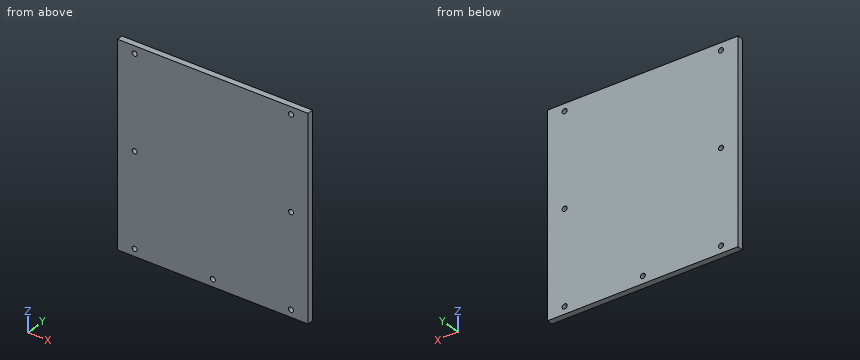
from build123d import *

# Parameters (mm, degrees)
SKETCH2_W           = 190.5
SKETCH2_H           = 203.2
BOSS_EXTRUDE1_DEPTH = 6
SKETCH5_R           = 2.5
CUT_EXTRUDE6_DEPTH  = 7


with BuildPart() as part:
    # Sketch2 → Boss-Extrude1 (new body)
    with BuildSketch(Plane(origin=(0, 0, 0), x_dir=(1, 0, 0), z_dir=(0, 1, 0))):
        Rectangle(SKETCH2_W, SKETCH2_H)
    extrude(amount=BOSS_EXTRUDE1_DEPTH)

    # Sketch5 → Cut-Extrude6 (cut, through all)
    with BuildSketch(Plane(origin=(0, 6, 0), x_dir=(1, 0, 0), z_dir=(0, 1, 0))):
        with Locations((-78.187036158, 94.165073798)):
            Circle(SKETCH5_R)
        with Locations((0, 94.165073798)):
            Circle(SKETCH5_R)
        with Locations((78.187036158, 0)):
            Circle(SKETCH5_R)
        with Locations((-78.187036158, 0)):
            Circle(SKETCH5_R)
        with Locations((78.187036158, 94.165073798)):
            Circle(SKETCH5_R)
        with Locations((-78.187036158, -94.165073798)):
            Circle(SKETCH5_R)
        with Locations((78.187036158, -94.165073798)):
            Circle(SKETCH5_R)
    extrude(amount=-CUT_EXTRUDE6_DEPTH, mode=Mode.SUBTRACT)


solid = part.part
For this review, take the finished solid that the model builds, in its own axes (mm). Give positions to 0.01 mm unless a question says otherwise; leave off trailing zeros. Order: outer loops, then holes, each group sorted by start corner. A loop starts at its lowest first (then second) coordinate and runs counter-clockwise, first axis right, second up. Notation, with made-up numbers: (36.5, 23) -> (80.5, 23) arc R15 cw to (80.5, 28) -> close; hole circle Ø8 at (74, 43). An arc over 180 degrees is marked (long way). Write item = value, one per line.
1) We need section B-B, the plane x = 0. Give the boundary of the cut face in (y, z).
Findings:
outline = (0, -101.6) -> (6, -101.6) -> (6, -96.67) -> (0, -96.67) -> close; (0, -91.67) -> (6, -91.67) -> (6, 101.6) -> (0, 101.6) -> close
2) We need section A-A, the plane z = 0. Give the boundary of the cut face in (x, y).
Findings:
outline = (-95.25, 0) -> (-80.69, 0) -> (-80.69, 6) -> (-95.25, 6) -> close; (-75.69, 0) -> (75.69, 0) -> (75.69, 6) -> (-75.69, 6) -> close; (80.69, 0) -> (95.25, 0) -> (95.25, 6) -> (80.69, 6) -> close
3) Insertion check: pin 1 (4.5 mm diameter, centred on x = 78.19, z = 94.17, fed in from +Y). The pin has a flat end and moves straight along its axis. Give the tip position at first contact, or say it passes through.
Findings:
pin_1 = through
4) To check wall thickness, follow L1, parallel to X at y = 3.85, z = 0; L2, parallel to Z at x = -77.5, y = 4.5; L3, parallel to Z at x = 1, y = 4.05. State the ranges of each line that lie inside material, in increasing order. Write a range as from..to.
Findings:
L1 = -95.25..-80.69, -75.69..75.69, 80.69..95.25
L2 = -101.6..-96.57, -91.76..-2.4, 2.4..91.76, 96.57..101.6
L3 = -101.6..-96.46, -91.87..101.6
